The listing builds one solid part. Answer for the finished solid, in the listing's coordinates (mm). Coordinates: 2 decimals unless noted, no trailing zeros. Order: outer loops, then holes, each group sorted by start corner. A loop starts at its lowest first (then second) coordinate and runs counter-clockwise, first axis right, second up. Notation, with made-up numbers: (46, -40) -> (103, -40) arc R3 ccw to (103, -36) -> close; hole circle Ø4 at (-26, 57.25). An arc over 180 degrees is marked (long way). Write item = value, one per line.
from build123d import *

# Parameters (mm, degrees)
SKETCH1_R           = 3
BOSS_EXTRUDE1_DEPTH = 15
CUT_EXTRUDE1_START  = -12
CUT_EXTRUDE1_DEPTH  = 12
SKETCH3_R           = 1.5
CUT_EXTRUDE2_DEPTH  = 6


with BuildPart() as part:
    # Sketch1 → Boss-Extrude1 (new body)
    with BuildSketch(Plane.XY):
        Circle(SKETCH1_R)
    extrude(amount=BOSS_EXTRUDE1_DEPTH)

    # Sketch2 → Cut-Extrude1 (cut)
    with BuildSketch(Plane.XY.offset(15).offset(CUT_EXTRUDE1_START)):
        with BuildLine():
            Line((-1.658312395, 2.5), (1.658312395, 2.5))
            ThreePointArc((1.658312395, 2.5), (0, 3), (-1.658312395, 2.5))
        make_face()
    extrude(amount=CUT_EXTRUDE1_DEPTH, mode=Mode.SUBTRACT)

    # Sketch3 → Cut-Extrude2 (cut)
    with BuildSketch(Plane(origin=(0, 2.5, 0), x_dir=(1, 0, 0), z_dir=(0, 1, 0))):
        with Locations(Location((0, -9, 0), (0, 0, 270))):
            Circle(SKETCH3_R)
    extrude(amount=-CUT_EXTRUDE2_DEPTH, mode=Mode.SUBTRACT)


solid = part.part
Q1. This flat-tipped pin is pushed along its axis until it touches: pin 1 Ø2 at (x, z) = (-2, 6) entering from +Y. Where does it stop, or does it pass through?
The answers:
pin_1 = 2.5
Q2. Section B-B, the plane y = -1 is taken. Give the vertices of the cut face in (x, z).
The answers:
outline = (-2.83, 0) -> (2.83, 0) -> (2.83, 15) -> (-2.83, 15) -> close; hole circle Ø3 at (0, 9)
Q3. Section D-D, the plane z = 6 is taken. Give the vertices of the cut face in (x, y).
The answers:
outline = (-1.66, 2.5) arc R3 ccw (long way) to (1.66, 2.5) -> close
Q4. Find the intervals of material crossed by line 1 along Z through (x, y) = (0, -0.8); line 2 along X through (y, z) = (0.65, 9); line 3 along X through (y, z) = (-1.3, 9), in increasing order.
The answers:
line_1 = 0 to 7.5, 10.5 to 15
line_2 = -2.93 to -1.5, 1.5 to 2.93
line_3 = -2.7 to -1.5, 1.5 to 2.7
Q5. The mould has two halves that part along X. Classify faces 1 (the face through (-0.575, -0.212, 10.386)), 2 (the face through (-0.65, -2.93, 7.4)), 3 (the face through (1.1, 2.5, 7.6)): released by +X, released by -X, zero draft, split by the parting line, or undercut.
The answers:
face_1 = undercut
face_2 = split by the parting line
face_3 = zero draft
Q6. Section C-C, the plane z = 9 is taken. Give the vertices of the cut face in (x, y), plus the area to 3 significant figures.
The answers:
outline = (-1.66, 2.5) arc R3 ccw to (-1.5, -2.6) -> (-1.5, 2.5) -> close; (1.5, -2.6) arc R3 ccw to (1.66, 2.5) -> (1.5, 2.5) -> close
area = 11.0 mm2
Q7. Section A-A, the plane x = 0 is taken. Give the vertices of the cut face in (y, z), plus the area to 3 significant figures.
The answers:
outline = (-3, 0) -> (3, 0) -> (3, 3) -> (2.5, 3) -> (2.5, 7.5) -> (-3, 7.5) -> close; (-3, 10.5) -> (2.5, 10.5) -> (2.5, 15) -> (-3, 15) -> close
area = 67.5 mm2
